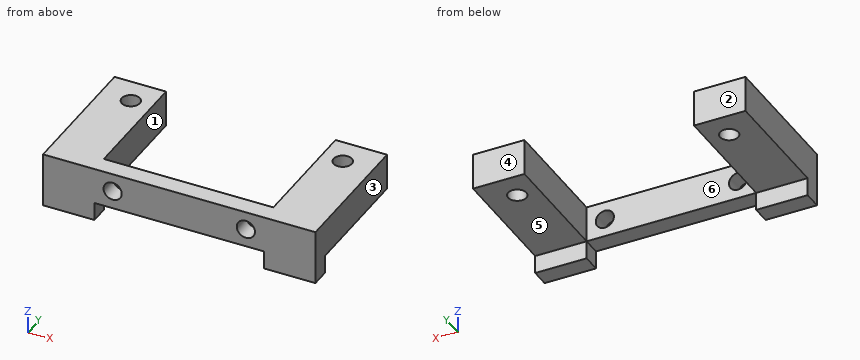
Autodesk Fusion 360 part; units mm, degrees
sketch "Sketch principal" plane through (0, 0, 0) normal (0, 0, 1) x (1, 0, 0)
  line L0 (45, 0) -> (45, 23)
  line L1 (45, 23) -> (36.5, 23)
  line L2 (36.5, 0) -> (45, 0)
  line L3 (36.5, 23) -> (36.5, 0)
  circle A0 centre (40, 18.5) radius 1.5
  line L4 (8.5, 23) -> (0, 23)
  line L5 (0, 0) -> (8.5, 0)
  line L6 (0, 23) -> (0, 0)
  line L7 (8.5, 0) -> (8.5, 23)
  circle A1 centre (5, 18.5) radius 1.5
  line L8 (8.5, 0) -> (36.5, 0)
  line L9 (36.5, 0) -> (36.5, 3)
  line L10 (36.5, 3) -> (8.5, 3)
  line L11 (8.5, 3) -> (8.5, 0)
  line L12 (8.5, 3) -> (0, 3)
  line L13 (0, 3) -> (0, 0)
  line L14 (0, 0) -> (8.5, 0)
  line L15 (8.5, 0) -> (8.5, 3)
  line L16 (36.5, 3) -> (45, 3)
  line L17 (45, 3) -> (45, 0)
  line L18 (45, 0) -> (36.5, 0)
  line L19 (36.5, 0) -> (36.5, 3)
  point P0 (36.5, 0)
  dimension "d15" = 23
  dimension "d16" = 8.5
  dimension "d17" = 3
  dimension "d18" = 4.5
  dimension "d20" = 23
  dimension "d21" = 8.5
  dimension "d22" = 3
  dimension "d23" = 4.5
  dimension "d24" = 3.5
  dimension "d25" = 28
  dimension "d26" = 3.5
  dimension "d28" = 3
  dimension "d29" = 28
extrude "Extrude1" add sketch "Sketch principal" along normal blind 6
ref_plane "WorkPlane1" through (22.5, 13, 3) normal (1, 0, 0) x (0, 1, 0)
ref_plane "WorkPlane2" through (22.5, 11.5, 3) normal (0, 0, -1) x (-1, 0, 0)
sketch "Sketch4" plane through (0, 3, 0) normal (0, 1, 0) x (-1, 0, 0)
  line L0 (-36.5, 0) -> (-8.5, 0)
  line L1 (-8.5, 0) -> (-8.5, 6)
  line L2 (-8.5, 6) -> (-36.5, 6)
  line L3 (-36.5, 6) -> (-36.5, 0)
  circle A0 centre (-11.5, 3) radius 1.5
  line L4 (-22.5, 0) -> (-22.5, 6)
  circle A1 centre (-33.5, 3) radius 1.5
  dimension "d32" = 3
  dimension "d35" = 3
extrude "Extrude2" cut sketch "Sketch4" against normal blind 11 contours A0 | A1
extrude "Extrude3" add sketch "Sketch principal" against normal blind 3 contours L0 L2 L3 L9 L16 L17 L18 L19 | L5 L6 L7 L11 L12 L13 L14 L15
The listing builds one solid part. Answer for the finished solid, in the listing's coordinates (mm). Face numbers are marked on the shaded views. A direction names the side the tool comes from. Round coordinates to 2 decimals unless told otherwise and drop trailing zeros. Loops run counter-clockwise (first coordinate to the right, second up) from the corner with the lowest first, then second, coordinate; pieces in that order, holes last. Notation, with made-up numbers: M -15.5,-8.75 L 42.5,-8.75 A28 ccw 42.5,18.25 Z; hole C 36.5,-37 d7. An arc over 180 degrees is marked long. Write each question's results on one line, items separated by ' | '. Start each with the question number.
1) Find section B-B on x = 33.5. Write down the section's boundary in (y, z), plus the area to 3 significant figures.
2) Which of the six approach directions +Z, -Z, +X, -X, +Y, -Y give full straight-line access (tool end or side, diameter ignored) to the marked faces 4, 5 and 6?
3) Straight lines are drawn through the part: probe 1 along X at (y, z) = (12.75, 5); probe 2 along Y at (x, z) = (5, 2.1); probe 3 along Y at (x, z) = (34, 0.5). For each, find the intervals that lie inside material, in ascending order.
4) Find section C-C on y = 18.5. Write down the section's boundary in (x, z), plus the area to 3 significant figures.
5) Find section D-D on y = 9.75. Write down the section's boundary in (x, z).
6) Find section A-A on z = 3. Write down the section's boundary in (x, y), plus the area to 3 significant figures.
7) Determine the mould class of the marked faces 1, 2 and 3 for opening direction X: pulls with the +X half, pulls with the -X half, needs draft (parallel to the pull), parting line crosses it, or undercut.
8) Each of these flat-tipped pins is pushed along its axis until it touches: pin 1 (9.5 mm diameter, centred on x = 4, y = 12, fed in from -Z); pin 2 (2.5 mm diameter, centred on x = 40, z = -1.5, fed in from +Y); pin 3 (1.8 mm diameter, centred on x = 5, y = 18.5, fed in from +Z). Where does it stop, or does it pass through?
Final values:
1) outline: M 0,0 L 3,0 L 3,1.5 L 0,1.5 Z; M 0,4.5 L 3,4.5 L 3,6 L 0,6 Z | area: 9.00 mm²
2) face 4: +Z, -Z, +X, -X, +Y | face 5: -Z, +X, -X, +Y | face 6: +Z, -Z, +Y
3) probe 1: 0 to 8.5, 36.5 to 45 | probe 2: 0 to 17, 20 to 23 | probe 3: 0 to 3
4) outline: M 0,0 L 3.5,0 L 3.5,6 L 0,6 Z; M 6.5,0 L 8.5,0 L 8.5,6 L 6.5,6 Z; M 36.5,0 L 38.5,0 L 38.5,6 L 36.5,6 Z; M 41.5,0 L 45,0 L 45,6 L 41.5,6 Z | area: 66.0 mm²
5) outline: M 0,0 L 8.5,0 L 8.5,6 L 0,6 Z; M 36.5,0 L 45,0 L 45,6 L 36.5,6 Z
6) outline: M 0,0 L 10,0 L 10,3 L 8.5,3 L 8.5,23 L 0,23 Z; M 13,0 L 32,0 L 32,3 L 13,3 Z; M 35,0 L 45,0 L 45,23 L 36.5,23 L 36.5,3 L 35,3 Z; hole C 5,18.5 d3; hole C 40,18.5 d3 | area: 443 mm²
7) face 1: undercut | face 2: needs draft | face 3: pulls with the +X half
8) pin 1: z = 0 | pin 2: y = 3 | pin 3: through
